Check sheet for the modelled part. Datum: model origin and axes. Units: mm. Face numbers are marked on the shaded views. Give positions to 0.01 mm unless a question says otherwise; leave off trailing zeros. Order: outer loops, then holes, each group sorted by start corner. A loop starts at its lowest first (then second) coordinate and runs counter-clockwise, first axis right, second up. Notation, with made-up numbers: M 14,63.5 L 57,63.5 A19 cw 57,89.5 Z; hole C 80,-37 d10. An arc over 180 degrees is marked long. Return JSON: item names as keys, results as strings. Group by question number.
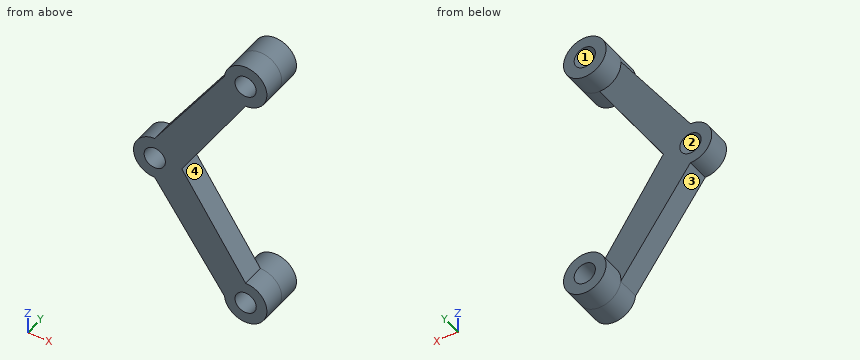
from build123d import *

# Parameters (mm, degrees)
SKETCH2_R           = 1.375
BOSS_EXTRUDE1_DEPTH = 3
SKETCH3_R           = 2.75
SKETCH3_R_2         = 1.375
BOSS_EXTRUDE2_DEPTH = 3


with BuildPart() as part:
    # Sketch2 → Boss-Extrude1 (new body)
    with BuildSketch(Plane(origin=(0, 0, 0), x_dir=(1, 0, 0), z_dir=(0, 1, 0))):
        with BuildLine():
            Line((-27, -2.75), (-17.987773433, -15.509030166))
            ThreePointArc((-17.987773433, -15.509030166), (-13.21593597, -17.100698117), (-15.25, -12.5))
            Line((-15.25, -12.5), (-23.5, 0))
            Line((-23.5, 0), (-15.25, 12.5))
            ThreePointArc((-15.25, 12.5), (-13.21593597, 17.100698117), (-17.987773433, 15.509030166))
            Line((-17.987773433, 15.509030166), (-27, 2.75))
            ThreePointArc((-27, 2.75), (-29.75, 0), (-27, -2.75))
        make_face()
        with Locations(Location((-27, 0, 0), (0, 0, 270))):
            Circle(SKETCH2_R, mode=Mode.SUBTRACT)
        with Locations(Location((-15.25, 15.25, 0), (0, 0, 270))):
            Circle(SKETCH2_R, mode=Mode.SUBTRACT)
        with Locations(Location((-15.25, -15.25, 0), (0, 0, 270))):
            Circle(SKETCH2_R, mode=Mode.SUBTRACT)
    extrude(amount=BOSS_EXTRUDE1_DEPTH)

    # Sketch3 → Boss-Extrude2 (add)
    # profile 1 of 2: a face of its own
    with BuildSketch(Plane(origin=(0, 3, 0), x_dir=(1, 0, 0), z_dir=(0, 1, 0))):
        with Locations(Location((-15.25, 15.25, 0), (0, 0, 270))):
            Circle(SKETCH3_R)
        with Locations(Location((-15.25, 15.25, 0), (0, 0, 270))):
            Circle(SKETCH3_R_2, mode=Mode.SUBTRACT)
    # profile 2 of 2: a face of its own
    with BuildSketch(Plane(origin=(0, 3, 0), x_dir=(1, 0, 0), z_dir=(0, 1, 0))):
        with Locations(Location((-15.25, -15.25, 0), (0, 0, 90))):
            Circle(SKETCH3_R)
        with Locations(Location((-15.25, -15.25, 0), (0, 0, 270))):
            Circle(SKETCH3_R_2, mode=Mode.SUBTRACT)
    extrude(amount=BOSS_EXTRUDE2_DEPTH)


solid = part.part
1) Sectioned sample at D-D on y = 4.15. Record the boundary of the cut face in (x, z) (3 decimals), then the cut area to 3 significant figures.
2) Depth check by flat-ended pin: P1, Ø2, axis at x = -27, z = 0, coming from the +Y side; P2, Ø1, axis at y = 1.5, z = -11.5, coming from the -X side; P3, Ø3, axis at x = -25.5, y = 1.5, coming from the +Z side; P4, Ø5, axis at x = -18.5, z = 7, coming from the +Y side. Enter the tip coordinate at first touch or a pass-through.
3) Release check for a two-part mould opening along X. For the marked faces 1, 2, 3 and 4 record: released by +X, released by -X, zero draft, split by the parting line, or undercut.
4) Material ranges on line 1 along Z through (x, y) = (-14.5, 1.35); line 2 along Z through (x, y) = (-15.75, 3.7); line 3 along X through (y, z) = (2.7, 15.25) (3 decimals), recorded low to high.
5) Sectioned sample at C-C on x = -18.5. Record the boundary of the cut face in (y, z).
6) Sectioned sample at B-B on x = -16. Record the boundary of the cut face in (y, z), then the cut area to 3 significant figures.
7) Sectioned sample at A-A on y = 0.9. Record the boundary of the cut face in (x, z) (3 decimals).
Reply:
{
 "1": {"outline": "C -15.25,-15.25 d5.5; C -15.25,15.25 d5.5; hole C -15.25,-15.25 d2.75; hole C -15.25,15.25 d2.75", "area": "35.6 mm^2"},
 "2": {"P1": "through", "P2": "x = -21.17", "P3": "z = 7", "P4": "y = 3"},
 "3": {"face 1": "undercut", "face 2": "undercut", "face 3": "released by -X", "face 4": "released by +X"},
 "4": {"line 1": "-17.9 to -16.4, -14.1 to -12.6, 12.6 to 14.1, 16.4 to 17.9", "line 2": "-17.95 to -16.53, -13.97 to -12.55, 12.55 to 13.97, 16.53 to 17.95", "line 3": "-18.171 to -16.625, -13.875 to -12.5"},
 "5": {"outline": "M 0,-14.78 L 3,-14.78 L 3,-7.58 L 0,-7.58 Z; M 0,7.58 L 3,7.58 L 3,14.78 L 0,14.78 Z"},
 "6": {"outline": "M 0,-17.9 L 6,-17.9 L 6,-16.4 L 0,-16.4 Z; M 0,-14.1 L 6,-14.1 L 6,-12.6 L 3,-12.6 L 3,-11.36 L 0,-11.36 Z; M 0,11.36 L 3,11.36 L 3,12.6 L 6,12.6 L 6,14.1 L 0,14.1 Z; M 0,16.4 L 6,16.4 L 6,17.9 L 0,17.9 Z", "area": "43.3 mm^2"},
 "7": {"outline": "M -27,-2.75 L -17.988,-15.509 A2.75 ccw long -15.25,-12.5 L -23.5,0 L -15.25,12.5 A2.75 ccw long -17.988,15.509 L -27,2.75 A2.75 ccw Z; hole C -27,0 d2.75; hole C -15.25,-15.25 d2.75; hole C -15.25,15.25 d2.75"}
}
